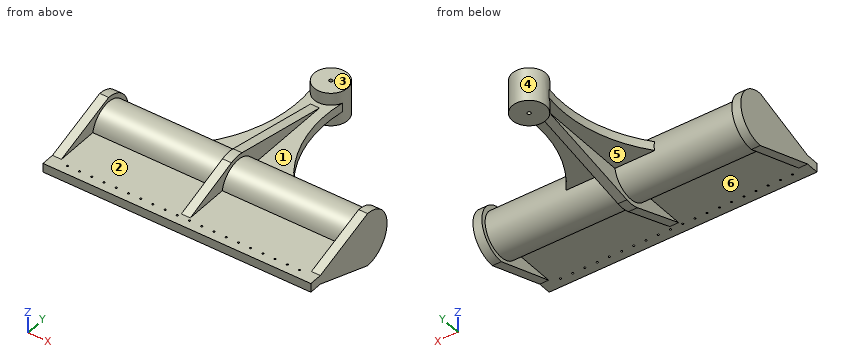
```python
from build123d import *

# Parameters (mm, degrees)
COEFFICIENTS_PLATE_DEPTH      = 2.54
COEFFICIENTS_PLATE_DEPTH_BACK = 2.54
COEFFICIENTS_PLATE_SKETCH_W   = 44.45
COEFFICIENTS_PLATE_SKETCH_H   = 152.4
COEFFICIENTS_PLATE_SKETCH_R   = 0.508
PIVOT_CYLINDER_DEPTH          = 76.2
PIVOT_CYLINDER_DEPTH_BACK     = 76.2
PIVOT_CYLINDER_SKETCH_R       = 12.7
EDGE_START                    = 71.12
EDGE_RIB_FRONT_DEPTH          = 5.08
EDGE_START_2                  = -76.2
EDGE_RIB_BACK_DEPTH           = 5.08
SUMMATION_PLATE_DEPTH         = 2.54
SUMMATION_PLATE_DEPTH_BACK    = 2.54
SUMMATION_ANCHOR_DEPTH        = 9.525
SUMMATION_ANCHOR_DEPTH_BACK   = 9.525
SUMMATION_ANCHOR_SKETCH_R     = 9.525
SUMMATION_ANCHOR_SKETCH_R_2   = 1.016
MIDDLE_RIB_DEPTH              = 2.54
MIDDLE_RIB_DEPTH_BACK         = 2.54


with BuildPart() as part:
    # Coefficients Plate Sketch → Coefficients Plate (new, two sides: drawn at the far end of the back side and taken through both)
    with BuildSketch(Plane(origin=(0, 0, 0), x_dir=(0, 1, 0), z_dir=(0, 0, 1)).offset(-COEFFICIENTS_PLATE_DEPTH_BACK)):
        with Locations((-22.225, 0)):
            Rectangle(COEFFICIENTS_PLATE_SKETCH_W, COEFFICIENTS_PLATE_SKETCH_H)
        with Locations(Location((-39.37, -66.04, 0), (0, 0, 270))):
            Circle(COEFFICIENTS_PLATE_SKETCH_R, mode=Mode.SUBTRACT)
        with Locations(Location((-39.37, -59.088421053, 0), (0, 0, 270))):
            Circle(COEFFICIENTS_PLATE_SKETCH_R, mode=Mode.SUBTRACT)
        with Locations(Location((-39.37, -52.136842105, 0), (0, 0, 270))):
            Circle(COEFFICIENTS_PLATE_SKETCH_R, mode=Mode.SUBTRACT)
        with Locations(Location((-39.37, -45.185263158, 0), (0, 0, 270))):
            Circle(COEFFICIENTS_PLATE_SKETCH_R, mode=Mode.SUBTRACT)
        with Locations(Location((-39.37, -38.233684211, 0), (0, 0, 270))):
            Circle(COEFFICIENTS_PLATE_SKETCH_R, mode=Mode.SUBTRACT)
        with Locations(Location((-39.37, -31.282105263, 0), (0, 0, 270))):
            Circle(COEFFICIENTS_PLATE_SKETCH_R, mode=Mode.SUBTRACT)
        with Locations(Location((-39.37, -24.330526316, 0), (0, 0, 270))):
            Circle(COEFFICIENTS_PLATE_SKETCH_R, mode=Mode.SUBTRACT)
        with Locations(Location((-39.37, -17.378947368, 0), (0, 0, 270))):
            Circle(COEFFICIENTS_PLATE_SKETCH_R, mode=Mode.SUBTRACT)
        with Locations(Location((-39.37, -10.427368421, 0), (0, 0, 270))):
            Circle(COEFFICIENTS_PLATE_SKETCH_R, mode=Mode.SUBTRACT)
        with Locations(Location((-39.37, -3.475789474, 0), (0, 0, 270))):
            Circle(COEFFICIENTS_PLATE_SKETCH_R, mode=Mode.SUBTRACT)
        with Locations(Location((-39.37, 3.475789474, 0), (0, 0, 270))):
            Circle(COEFFICIENTS_PLATE_SKETCH_R, mode=Mode.SUBTRACT)
        with Locations(Location((-39.37, 10.427368421, 0), (0, 0, 270))):
            Circle(COEFFICIENTS_PLATE_SKETCH_R, mode=Mode.SUBTRACT)
        with Locations(Location((-39.37, 17.378947368, 0), (0, 0, 270))):
            Circle(COEFFICIENTS_PLATE_SKETCH_R, mode=Mode.SUBTRACT)
        with Locations(Location((-39.37, 24.330526316, 0), (0, 0, 270))):
            Circle(COEFFICIENTS_PLATE_SKETCH_R, mode=Mode.SUBTRACT)
        with Locations(Location((-39.37, 31.282105263, 0), (0, 0, 270))):
            Circle(COEFFICIENTS_PLATE_SKETCH_R, mode=Mode.SUBTRACT)
        with Locations(Location((-39.37, 38.233684211, 0), (0, 0, 270))):
            Circle(COEFFICIENTS_PLATE_SKETCH_R, mode=Mode.SUBTRACT)
        with Locations(Location((-39.37, 45.185263158, 0), (0, 0, 270))):
            Circle(COEFFICIENTS_PLATE_SKETCH_R, mode=Mode.SUBTRACT)
        with Locations(Location((-39.37, 52.136842105, 0), (0, 0, 270))):
            Circle(COEFFICIENTS_PLATE_SKETCH_R, mode=Mode.SUBTRACT)
        with Locations(Location((-39.37, 59.088421053, 0), (0, 0, 270))):
            Circle(COEFFICIENTS_PLATE_SKETCH_R, mode=Mode.SUBTRACT)
        with Locations(Location((-39.37, 66.04, 0), (0, 0, 270))):
            Circle(COEFFICIENTS_PLATE_SKETCH_R, mode=Mode.SUBTRACT)
    extrude(amount=COEFFICIENTS_PLATE_DEPTH + COEFFICIENTS_PLATE_DEPTH_BACK)

    # Pivot Cylinder Sketch → Pivot Cylinder (add, two sides: drawn at the far end of the back side and taken through both)
    with BuildSketch(Plane.YZ.offset(-PIVOT_CYLINDER_DEPTH_BACK)):
        Circle(PIVOT_CYLINDER_SKETCH_R)
    extrude(amount=PIVOT_CYLINDER_DEPTH + PIVOT_CYLINDER_DEPTH_BACK)

    # Edge Rib Front Sketch → Edge Rib Front (add)
    with BuildSketch(Plane.YZ.offset(EDGE_START)):
        with BuildLine():
            Line((0, 15.24), (-44.45, 0))
            Line((-44.45, 0), (0, -15.24))
            ThreePointArc((0, -15.24), (15.24, 0), (0, 15.24))
        make_face()
    extrude(amount=EDGE_RIB_FRONT_DEPTH)

    # Edge Rib Back Sketch → Edge Rib Back (add)
    with BuildSketch(Plane.YZ.offset(EDGE_START_2)):
        with BuildLine():
            Line((0, 15.24), (-44.45, 0))
            Line((-44.45, 0), (0, -15.24))
            ThreePointArc((0, -15.24), (15.24, 0), (0, 15.24))
        make_face()
    extrude(amount=EDGE_RIB_BACK_DEPTH)

    # Summation Plate Sketch → Summation Plate (add, two sides: drawn at the far end of the back side and taken through both)
    with BuildSketch(Plane(origin=(0, 0, 0), x_dir=(0, 1, 0), z_dir=(0, 0, 1)).offset(-SUMMATION_PLATE_DEPTH_BACK)):
        with BuildLine():
            Line((0, -38.1), (0, 38.1))
            ThreePointArc((0, 38.1), (33.985630195, 12.840847186), (76.2, 9.525))
            Line((76.2, 9.525), (76.2, -9.525))
            ThreePointArc((76.2, -9.525), (33.985630195, -12.840847186), (0, -38.1))
        make_face()
    extrude(amount=SUMMATION_PLATE_DEPTH + SUMMATION_PLATE_DEPTH_BACK)

    # Summation Anchor Sketch → Summation Anchor (add, two sides: drawn at the far end of the back side and taken through both)
    with BuildSketch(Plane(origin=(0, 0, 0), x_dir=(0, 1, 0), z_dir=(0, 0, 1)).offset(-SUMMATION_ANCHOR_DEPTH_BACK)):
        with Locations(Location((76.2, 0, 0), (0, 0, 270))):
            Circle(SUMMATION_ANCHOR_SKETCH_R)
        with Locations(Location((76.2, 0, 0), (0, 0, 270))):
            Circle(SUMMATION_ANCHOR_SKETCH_R_2, mode=Mode.SUBTRACT)
    extrude(amount=SUMMATION_ANCHOR_DEPTH + SUMMATION_ANCHOR_DEPTH_BACK)

    # Middle Rib Sketch → Middle Rib (add, two sides: drawn at the far end of the back side and taken through both)
    with BuildSketch(Plane.YZ.offset(-MIDDLE_RIB_DEPTH_BACK)):
        with BuildLine():
            Line((-44.45, 0), (-5.225026376, 14.316255211))
            ThreePointArc((-5.225026376, 14.316255211), (-1.131177872, 15.197936065), (3.048089123, 14.93207128))
            Line((3.048089123, 14.93207128), (76.2, 0))
            Line((76.2, 0), (3.048089123, -14.93207128))
            ThreePointArc((3.048089123, -14.93207128), (-1.131177872, -15.197936065), (-5.225026376, -14.316255211))
            Line((-5.225026376, -14.316255211), (-44.45, 0))
        make_face()
    extrude(amount=MIDDLE_RIB_DEPTH + MIDDLE_RIB_DEPTH_BACK)


solid = part.part
```
The listing builds one solid part. Answer for the finished solid, in the listing's coordinates (mm). Face numbers are marked on the shaded views. A direction names the side the tool comes from. Give positions to 0.01 mm unless a question says otherwise; leave off trailing zeros. Order: outer loops, then holes, each group sorted by start corner. A loop starts at its lowest first (then second) coordinate and runs counter-clockwise, first axis right, second up. Notation, with made-up numbers: (82, 77) - (119, 77) arc R28 ccw to (119, 99) - close; hole circle Ø10 at (30.5, 26.5). An arc over 180 degrees is marked (long way). Use one line per item in the form item = value. Start each with the question number.
(1) A cutting plane is placed at C-C, the plane x = -41. Write down the section's boundary in (y, z), then the cut area to 3 significant figures.
(2) A cutting plane is placed at A-A, the plane z = -6.5. Write down the section's boundary in (x, y) (3 decimals), then the cut area to 3 significant figures.
(3) Flat-ended cylindrical pins translate along their axes: pin 1 Ø0.9 at (x, y) = (-10.43, -39.37) entering from +Z; pin 2 Ø25 at (x, y) = (5.5, 47) entering from -Z; pin 3 Ø8 at (x, z) = (-14, -9.5) entering from -Y; pin 4 Ø4 at (x, z) = (-18.5, -10) entering from +Y. Find the tip coordinate at first contact, or state that the pin passes through.
(4) The mould has two halves that part along Y. Classify the marked faces 5 and 6: released by +Y, released by -Y, zero draft, split by the parting line, or undercut.
(5) Consider line 1 (X direction, y = -18, z = -6.5); line 2 (Y direction, x = 66, z = 0); line 3 (X direction, y = 21, z = -3). Determine where each line is inside the solid, lowest interval first. Write a range as from..to.
(6) A cutting plane is placed at B-B, the plane y = 69. Write down the section's boundary in (x, z) (3 decimals).
(7) For the marked faces 1, 2, 3 and 4, determine the directions among +Z, -Z, +X, -X, +Y, -Y from which every point of the face is accessible in a straight line to the end or side of a thin tool.
(8) A cutting plane is placed at D-D, the plane x = -13. Write down the section's boundary in (y, z).
Ans:
q1.outline = (-44.45, -2.54) - (-12.44, -2.54) arc R12.7 ccw (long way) to (-12.44, 2.54) - (-44.45, 2.54) - close
q1.area = 668 mm^2
q2.outline = (-76.2, -25.492) - (-71.12, -25.492) - (-71.12, -10.911) - (-2.54, -10.911) - (-2.54, -26.641) - (2.54, -26.641) - (2.54, -10.911) - (71.12, -10.911) - (71.12, -25.492) - (76.2, -25.492) - (76.2, 13.784) - (71.12, 13.784) - (71.12, 10.911) - (2.54, 10.911) - (2.54, 44.357) - (-2.54, 44.357) - (-2.54, 10.911) - (-71.12, 10.911) - (-71.12, 13.784) - (-76.2, 13.784) - close; circle Ø19.05 at (0, 76.2); hole circle Ø2.032 at (0, 76.2)
q2.area = 4,030 mm^2
q3.pin_1 = through
q3.pin_2 = -8.44
q3.pin_3 = -11.45
q3.pin_4 = 9.86
q4.face_5 = undercut
q4.face_6 = zero draft
q5.line_1 = -76.2..-71.12, -2.54..2.54, 71.12..76.2
q5.line_2 = -44.45..-39.88, -38.86..12.7
q5.line_3 = -2.54..2.54
q6.outline = (-8.405, -2.54) - (-6.236, -2.54) - (-6.236, -9.525) - (6.236, -9.525) - (6.236, -2.54) - (8.405, -2.54) - (8.405, 2.54) - (6.236, 2.54) - (6.236, 9.525) - (-6.236, 9.525) - (-6.236, 2.54) - (-8.405, 2.54) - close
q7.face_1 = +Z
q7.face_2 = +Z, -Y
q7.face_3 = +Z, +X, -X, +Y
q7.face_4 = none
q8.outline = (-44.45, -2.54) - (-12.44, -2.54) arc R12.7 ccw to (12.44, -2.54) - (33.56, -2.54) - (33.56, 2.54) - (12.44, 2.54) arc R12.7 ccw to (-12.44, 2.54) - (-44.45, 2.54) - close
